from build123d import *

# Parameters (mm, degrees)
F1_DEPTH = 3
F2_DEPTH = 3
F4_DEPTH = 3
F6_R     = 11.5
F7_DEPTH = 2.6


with BuildPart() as f1:
    # F0 (on Front) → F1 (new body)
    with BuildSketch(Plane.XZ):
        with BuildLine():
            ThreePointArc((-7.4157768365, 6.7086700553), (-3.5945953621, -9.331606731), (10, 0))
            ThreePointArc((10, 0), (9.331606731, 3.5945953621), (7.4157768365, 6.7086700553))
            Line((7.4157768365, 6.7086700553), (5.6450560127, 4.9379492315))
            ThreePointArc((5.6450560127, 4.9379492315), (7.0209657489, 2.6374305588), (7.5, 0))
            ThreePointArc((7.5, 0), (-2.6374305588, -7.0209657489), (-5.6450560127, 4.9379492315))
            Line((-5.6450560127, 4.9379492315), (-7.4157768365, 6.7086700553))
        make_face()
    extrude(amount=F1_DEPTH)

    # F3 (on Front) → F4 (join, through all)
    with BuildSketch(Plane.XZ):
        with BuildLine():
            Line((-1.9912281105, -0.2941718356), (-6.0835066474, -4.3864503726))
            ThreePointArc((-6.0835066474, -4.3864503726), (-5.7118298294, -4.8605555238), (-5.3033008589, -5.3033008589))
            Line((-5.3033008589, -5.3033008589), (-0.5, -0.5))
            Line((-0.5, -0.5), (-0.5, 1.1970562748))
            Line((-0.5, 1.1970562748), (-1.9912281105, -0.2941718356))
        make_face()
        with BuildLine():
            Line((-0.5, -0.5), (-5.3033008589, -5.3033008589))
            ThreePointArc((-5.3033008589, -5.3033008589), (-4.8605555238, -5.7118298294), (-4.3864503726, -6.0835066474))
            Line((-4.3864503726, -6.0835066474), (-0.5, -2.1970562748))
            Line((-0.5, -2.1970562748), (-0.5, -0.5))
        make_face()
        Polygon((-0.5, 3.8029437252), (-1.9912281105, -0.2941718356), (-0.5, 1.1970562748), align=None)
        with BuildLine():
            Line((0.5, -0.5), (5.3033008589, -5.3033008589))
            ThreePointArc((5.3033008589, -5.3033008589), (5.7118298294, -4.8605555238), (6.0835066474, -4.3864503726))
            Line((6.0835066474, -4.3864503726), (1.9912281105, -0.2941718356))
            Line((1.9912281105, -0.2941718356), (0.5, 1.1970562748))
            Line((0.5, 1.1970562748), (0.5, -0.5))
        make_face()
        with BuildLine():
            Line((0.5, -2.1970562748), (4.3864503726, -6.0835066474))
            ThreePointArc((4.3864503726, -6.0835066474), (4.8605555238, -5.7118298294), (5.3033008589, -5.3033008589))
            Line((5.3033008589, -5.3033008589), (0.5, -0.5))
            Line((0.5, -0.5), (0.5, -2.1970562748))
        make_face()
        Polygon((0.5, 3.8029437252), (0.5, 1.1970562748), (1.9912281105, -0.2941718356), align=None)
    extrude(amount=F4_DEPTH)



with BuildPart() as f2:
    # F0 (on Front) → F2 (new body, through all)
    with BuildSketch(Plane.XZ):
        with BuildLine():
            Line((4.9379492315, 5.6450560127), (6.7086700553, 7.4157768365))
            ThreePointArc((6.7086700553, 7.4157768365), (0, 10), (-6.7086700553, 7.4157768365))
            Line((-6.7086700553, 7.4157768365), (-4.9379492315, 5.6450560127))
            ThreePointArc((-4.9379492315, 5.6450560127), (0, 7.5), (4.9379492315, 5.6450560127))
        make_face()
    extrude(amount=F2_DEPTH)


with BuildPart() as f1_1:
    add(f1.part)

    add(f2.part)  # F7 merges F2
    # F6 (on offset) → F7 (join)
    with BuildSketch(Plane(origin=(0, -0.2, 0), x_dir=(-1, 0, 0), z_dir=(0, 1, 0))):
        Circle(F6_R)
    extrude(amount=-F7_DEPTH)


solid = f1_1.part
Input: part model. Units: mm. Frame: model coordinates. Give positions to 0.01 mm unless a question says otherwise; leave off trailing zeros. Write each loop counter-clockwise with the first axis right and the second up, starting at its lowest first coordinate (ties: lowest second). Pieces come first, ordered by that corner, then holes. Notation, with made-up numbers: M 29,-30 L 56,-30 A21 ccw 56,9 Z; hole C 12,-18.5 d11. An arc over 180 degrees is marked long. Write item = value, one per line. Start each with the question number.
1) First-contact query: pin 1 Ø2 at (x, z) = (7, -9) entering from +Y; pin 2 Ø1 at (x, y) = (-1.5, -2) entering from -Z; pin 3 Ø1 at (x, y) = (-2, -0.5) entering from -Z. Flat tips, straight axial feed; report the tip coordinate or a pass-through.
2) Cut plane A-A on x = 0. Return the cut outline in (y, z), then the cut area to 3 significant figures.
3) Cut plane B-B on z = 8.75. Return the cut outline in (x, y).
4) Cut plane D-D on x = 3.5. Return the cut outline in (y, z).
5) Cut plane C-C on y = -1.2. Return the cut outline in (x, z), then the cut area to 3 significant figures.
6) Material intervals for line 1 along Y through (x, z) = (6.25, 9); line 2 along Z through (x, y) = (0, -2.75); line 3 along X through (y, z) = (-1.15, -3.75), sorted ascending. Write a range as [from, to].
7) Draft query along X for faces 1 (the flat face through (0, -0.2, 0)), 2 (the flat face through (-2, 0, -3)). Return one class per face: +X half, -X half, draft (parallel to the pull), parting line (faces both ways), or undercut.
Solved:
q1.pin_1 = -0.2
q1.pin_2 = -11.46
q1.pin_3 = -11.4
q2.outline = M -3,-10 L -2.8,-10 L -2.8,-11.5 L -0.2,-11.5 L -0.2,-10 L 0,-10 L 0,-7.5 L -0.2,-7.5 L -0.2,7.5 L 0,7.5 L 0,10 L -0.2,10 L -0.2,11.5 L -2.8,11.5 L -2.8,10 L -3,10 L -3,7.5 L -2.8,7.5 L -2.8,-7.5 L -3,-7.5 Z
q2.area = 61.8 mm2
q3.outline = M -7.46,-2.8 L -4.84,-2.8 L -4.84,-3 L 4.84,-3 L 4.84,-2.8 L 7.46,-2.8 L 7.46,-0.2 L 4.84,-0.2 L 4.84,0 L -4.84,0 L -4.84,-0.2 L -7.46,-0.2 Z
q4.outline = M -3,-9.37 L -2.8,-9.37 L -2.8,-10.95 L -0.2,-10.95 L -0.2,-9.37 L 0,-9.37 L 0,-6.63 L -0.2,-6.63 L -0.2,-5.2 L 0,-5.2 L 0,-1.8 L -0.2,-1.8 L -0.2,6.63 L 0,6.63 L 0,9.37 L -0.2,9.37 L -0.2,10.95 L -2.8,10.95 L -2.8,9.37 L -3,9.37 L -3,6.63 L -2.8,6.63 L -2.8,-1.8 L -3,-1.8 L -3,-5.2 L -2.8,-5.2 L -2.8,-6.63 L -3,-6.63 Z
q5.outline = C 0,0 d23
q5.area = 415 mm2
q6.line_1 = [-2.8, -0.2]
q6.line_2 = [-11.5, 11.5]
q6.line_3 = [-10.87, 10.87]
q7.face_1 = undercut
q7.face_2 = draft
